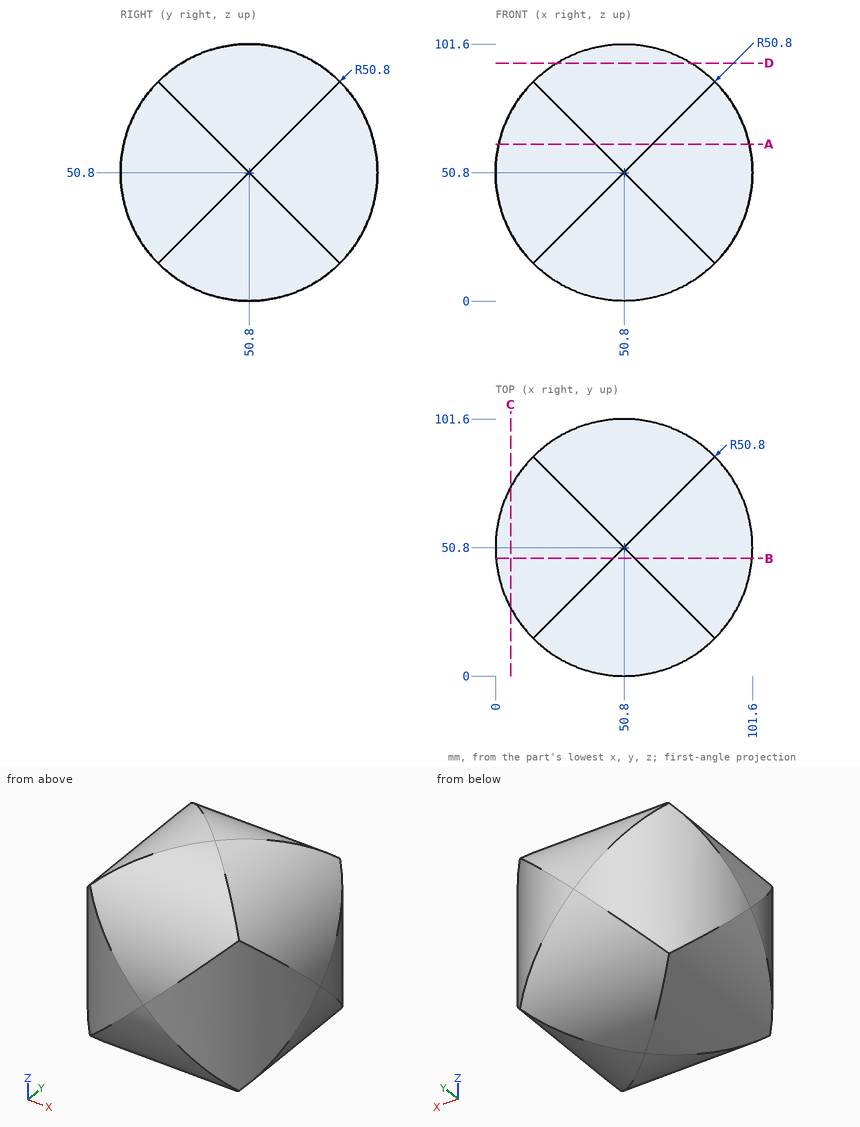
Geometry check sheet. Reference: drawing and pictorial views, mm from the part's lowest x, y, z. Round coordinates to 2 decimals unless told otherwise and drop trailing zeros. Write each loop counter-clockwise with the first axis right and the second up, starting at its lowest first coordinate (ties: lowest second). Pieces come first, ordered by that corner, then holes. Notation, with made-up numbers: (40, 32) -> (60, 32) arc R27 cw to (60, 51) -> close; hole circle Ø2 at (-5.75, 19.25). An arc over 180 degrees is marked (long way). One line per question, with ' | ' between items. Start each with the question number.
1. Sectioned sample at D-D, the plane z = 94. Record the cut outline in (x, y), then the cut area to 3 significant figures.
2. Sectioned sample at C-C, the plane x = 6. Record the cut outline in (y, z), then the cut area to 3 significant figures.
3. Sectioned sample at B-B, the plane y = 46.5. Record the cut outline in (x, z).
4. Depth check by flat-ended pin: pin 1 (10 mm diameter, centred on x = 13.5, z = 52.5, fed in from -Y); pin 2 (8 mm diameter, centred on y = 71, z = 59.5, fed in from +X); pin 3 (12 mm diameter, centred on x = 20.5, z = 59, fed in from -Y). Enter the tip coordinate at first touch or a pass-through.
5. Sectioned sample at A-A, the plane z = 62. Record the cut outline in (x, y), then the cut area to 3 significant figures.
6. Scan lines: line 1 along X through (y, z) = (63, 54); line 2 along Y through (x, z) = (53.5, 97); line 3 along Z through (x, y) = (39.5, 56). Record each from-to range of solid material in increasing order. Write a range as from..to.
Taken from the geometry:
1) outline: (24.07, 24.07) -> (77.53, 24.07) -> (77.53, 77.53) -> (24.07, 77.53) -> close | area: 2,860 mm^2
2) outline: (26.85, 26.85) -> (74.75, 26.85) -> (74.75, 74.75) -> (26.85, 74.75) -> close | area: 2,290 mm^2
3) outline: (0.18, 46.5) arc R50.8 ccw to (46.5, 0.18) -> (55.1, 0.18) arc R50.8 ccw to (101.42, 46.5) -> (101.42, 55.1) arc R50.8 ccw to (55.1, 101.42) -> (46.5, 101.42) arc R50.8 ccw to (0.18, 55.1) -> close
4) pin 1: stops at y = 11.59 | pin 2: stops at x = 98.95 | pin 3: stops at y = 6.19
5) outline: (1.25, 39.6) arc R50.8 ccw to (39.6, 1.25) -> (62, 1.25) arc R50.8 ccw to (100.35, 39.6) -> (100.35, 62) arc R50.8 ccw to (62, 100.35) -> (39.6, 100.35) arc R50.8 ccw to (1.25, 62) -> close | area: 8,030 mm^2
6) line 1: x = 1.49..100.11 | line 2: y = 29.68..71.92 | line 3: z = 1.27..100.33
